```python
from build123d import *

# Parameters (mm, degrees)
SKETCH11_R          = 3.96875
SKETCH11_R_2        = 15.08125
SKETCH11_R_3        = 2
BOSS_EXTRUDE2_DEPTH = 5.08


with BuildPart() as part:
    # Sketch11 → Boss-Extrude2 (new body)
    with BuildSketch(Plane(origin=(0, 0, 0), x_dir=(1, 0, 0), z_dir=(0, 1, 0))):
        with BuildLine():
            Line((19.05, -173.758834345), (19.05, -72.598586407))
            ThreePointArc((19.05, -72.598586407), (19.041478453, -72.390699795), (19.015970989, -72.184208077))
            Line((19.015970989, -72.184208077), (6.891420221, 1.139540409))
            ThreePointArc((6.891420221, 1.139540409), (0.187396777, 6.982485764), (-6.820377584, 1.507539257))
            Line((-6.820377584, 1.507539257), (-25.340137303, -82.279170439))
            ThreePointArc((-25.340137303, -82.279170439), (-25.384989975, -82.551639086), (-25.4, -82.827366533))
            Line((-25.4, -82.827366533), (-25.4, -177.8))
            Line((-25.4, -177.8), (-25.4, -228.6))
            ThreePointArc((-25.4, -228.6), (-22.745272537, -232.230626029), (-18.480606107, -230.801765114))
            Line((-18.480606107, -230.801765114), (16.71464631, -181.098051393))
            ThreePointArc((16.71464631, -181.098051393), (18.452086765, -177.609742801), (19.05, -173.758834345))
        make_face()
        Circle(SKETCH11_R, mode=Mode.SUBTRACT)
        with Locations((0, -160.246508934)):
            Circle(SKETCH11_R_2, mode=Mode.SUBTRACT)
        with Locations((-20.32, -225.425)):
            Circle(SKETCH11_R_3, mode=Mode.SUBTRACT)
        with Locations((-20.32, -219.075)):
            Circle(SKETCH11_R_3, mode=Mode.SUBTRACT)
        with Locations((-20.32, -212.725)):
            Circle(SKETCH11_R_3, mode=Mode.SUBTRACT)
        with Locations((-20.32, -206.375)):
            Circle(SKETCH11_R_3, mode=Mode.SUBTRACT)
        with Locations((0, -16.51)):
            Circle(SKETCH11_R_3, mode=Mode.SUBTRACT)
        with Locations((14.605, -176.756508934)):
            Circle(SKETCH11_R_3, mode=Mode.SUBTRACT)
        with BuildLine():
            Line((11.940278596, -80.334093652), (-14.464036902, -109.837128051))
            ThreePointArc((-14.464036902, -109.837128051), (-17.263416449, -110.515885849), (-18.896731016, -108.143224574))
            Line((-18.896731016, -108.143224574), (-18.896731016, -82.827366533))
            ThreePointArc((-18.896731016, -82.827366533), (-18.881720992, -82.551639086), (-18.83686832, -82.279170439))
            Line((-18.83686832, -82.279170439), (-6.80244992, -27.833306339))
            ThreePointArc((-6.80244992, -27.833306339), (-0.402909414, -22.833553189), (5.719243979, -28.169365038))
            Line((5.719243979, -28.169365038), (13.473470783, -75.063389134))
            ThreePointArc((13.473470783, -75.063389134), (13.305815609, -77.87296697), (11.940278596, -80.334093652))
        make_face(mode=Mode.SUBTRACT)
        with BuildLine():
            Line((13.97, -141.812492878), (13.97, -90.426050798))
            ThreePointArc((13.97, -90.426050798), (12.336685433, -88.053389523), (9.537305885, -88.732147321))
            Line((9.537305885, -88.732147321), (-15.843545445, -117.091607347))
            ThreePointArc((-15.843545445, -117.091607347), (-16.487420873, -118.917476564), (-15.657551613, -120.666673802))
            Line((-15.657551613, -120.666673802), (9.723299718, -143.693655856))
            ThreePointArc((9.723299718, -143.693655856), (12.458732541, -144.134842843), (13.97, -141.812492878))
        make_face(mode=Mode.SUBTRACT)
        with BuildLine():
            Line((-13.279299718, -127.111337727), (-2.809524218, -136.610125984))
            ThreePointArc((-2.809524218, -136.610125984), (-2.003545388, -138.86283126), (-3.426980373, -140.785879825))
            Line((-3.426980373, -140.785879825), (-13.896755873, -145.755890669))
            ThreePointArc((-13.896755873, -145.755890669), (-16.343372447, -145.60819059), (-17.526, -143.461299805))
            Line((-17.526, -143.461299805), (-17.526, -128.992500705))
            ThreePointArc((-17.526, -128.992500705), (-16.014732541, -126.67015074), (-13.279299718, -127.111337727))
        make_face(mode=Mode.SUBTRACT)
        with BuildLine():
            Line((6.282161105, -189.238159376), (-2.779804772, -202.035719466))
            ThreePointArc((-2.779804772, -202.035719466), (-6.184281083, -204.125642303), (-10.047215475, -203.107814076))
            Line((-10.047215475, -203.107814076), (-17.09155218, -197.621171408))
            ThreePointArc((-17.09155218, -197.621171408), (-18.534202289, -195.843739158), (-19.05, -193.613389978))
            Line((-19.05, -193.613389978), (-19.05, -183.748869713))
            ThreePointArc((-19.05, -183.748869713), (-17.268890157, -179.885746141), (-13.174518217, -178.731538875))
            Line((-13.174518217, -178.731538875), (2.931784364, -181.28514172))
            ThreePointArc((2.931784364, -181.28514172), (6.817844364, -184.330274157), (6.282161105, -189.238159376))
        make_face(mode=Mode.SUBTRACT)
        with BuildLine():
            Line((3.834506832, -6.35), (-3.834506832, -6.35))
            ThreePointArc((-3.834506832, -6.35), (-4.629741225, -6.629796859), (-5.074575483, -7.345901953))
            Line((-5.074575483, -7.345901953), (-5.636003302, -9.885901953))
            ThreePointArc((-5.636003302, -9.885901953), (-5.386137791, -10.955234393), (-4.395934651, -11.43))
            Line((-4.395934651, -11.43), (4.254512077, -11.43))
            ThreePointArc((4.254512077, -11.43), (5.223023884, -10.981513774), (5.507497571, -9.952810835))
            Line((5.507497571, -9.952810835), (5.087492326, -7.412810835))
            ThreePointArc((5.087492326, -7.412810835), (4.656020605, -6.651488193), (3.834506832, -6.35))
        make_face(mode=Mode.SUBTRACT)
    extrude(amount=-BOSS_EXTRUDE2_DEPTH)


solid = part.part
```
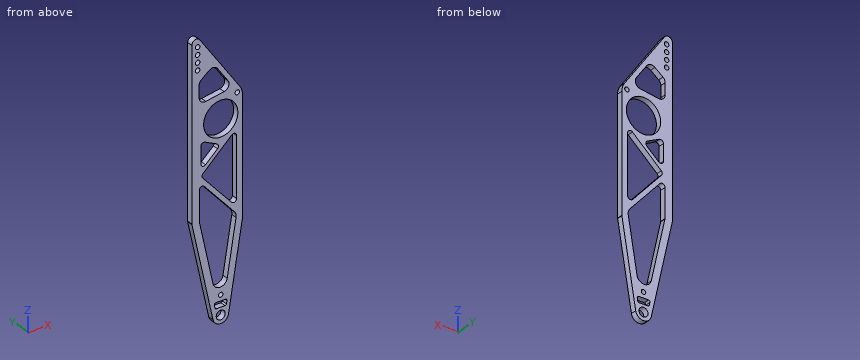
The listing builds one solid part. Answer for the finished solid, in the listing's coordinates (mm). Coordinates: 2 decimals unless noted, no trailing zeros. Order: outer loops, then holes, each group sorted by start corner. A loop starts at its lowest first (then second) coordinate and runs counter-clockwise, first axis right, second up. Notation, with made-up numbers: M 67.5,69.25 L 91.5,69.25 A13 cw 91.5,77.25 Z; hole C -19,-17 d10. An arc over 180 degrees is marked long. Answer as a JSON object with one key per item and string values. Group by question number.
1. Section B-B on x = 0 is taken. State how many separate pieces and enclosed holes the cut face has, then the cut area to 3 significant figures.
2. Flat-ended cylindrical pins translate along their axes: P1, Ø3.5, axis at x = -20.32, z = 219.075, coming from the -Y side; P2, Ø5, axis at x = 14.6, z = 176.76, coming from the -Y side; P3, Ø3, axis at y = -4.5, z = 67.5, coming from the +X side; P4, Ø1.5, axis at x = 1.5, y = -2, coming from the +Z side. Find the tip coordinate at first contact, or state that the pin passes through.
3. Section A-A on z = 16.51 is taken. Write down the section's boundary in (x, y).
4. Straight lines are drawn through the part: line 1 (X direction, y = -2.9, z = 86); line 2 (X direction, y = -0.5, z = 135); line 3 (X direction, y = -0.8, z = 98). For each, find the intervals that lie inside material, in ascending order.
Values follow:
{
 "1": {"separate pieces": "8", "enclosed holes": "0", "area": "208 mm2"},
 "2": {"P1": "through", "P2": "y = -5.08", "P3": "x = 18.49", "P4": "z = 203.64"},
 "3": {"outline": "M -10.8,-5.08 L -2,-5.08 L -2,0 L -10.8,0 Z; M 2,-5.08 L 9.81,-5.08 L 9.81,0 L 2,0 Z"},
 "4": {"line 1": "-25.4 to -18.9, 6.87 to 19.05", "line 2": "-25.4 to -17.53, -4.58 to 0.14, 13.97 to 19.05", "line 3": "-25.4 to -18.9, -3.87 to 1.24, 13.97 to 19.05"}
}
